```python
from build123d import *

# Parameters (mm, degrees)
SKETCH2_W           = 50
SKETCH2_H           = 53
BOSS_EXTRUDE1_DEPTH = 3
SKETCH3_W           = 50
SKETCH3_H           = 48
SKETCH3_R           = 11
BOSS_EXTRUDE2_DEPTH = 3
BOSS_EXTRUDE3_DEPTH = 3


with BuildPart() as part:
    # Sketch2 → Boss-Extrude1 (new body)
    with BuildSketch(Plane(origin=(0, 0, 0), x_dir=(1, 0, 0), z_dir=(0, 1, 0))):
        with Locations((25, 26.5)):
            Rectangle(SKETCH2_W, SKETCH2_H)
        with BuildLine():
            Line((7.9, 12), (7.9, 42))
            ThreePointArc((7.9, 42), (10, 44.1), (12.1, 42))
            Line((12.1, 42), (12.1, 12))
            ThreePointArc((12.1, 12), (10, 9.9), (7.9, 12))
        make_face(mode=Mode.SUBTRACT)
        with BuildLine():
            Line((42.1, 12), (42.1, 42))
            ThreePointArc((42.1, 42), (40, 44.1), (37.9, 42))
            Line((37.9, 42), (37.9, 12))
            ThreePointArc((37.9, 12), (40, 9.9), (42.1, 12))
        make_face(mode=Mode.SUBTRACT)
    extrude(amount=BOSS_EXTRUDE1_DEPTH)

    # Sketch3 → Boss-Extrude2 (add)
    with BuildSketch(Plane.XY):
        with Locations((25, 27)):
            Rectangle(SKETCH3_W, SKETCH3_H)
        with Locations((25, 30)):
            Circle(SKETCH3_R, mode=Mode.SUBTRACT)
    extrude(amount=-BOSS_EXTRUDE2_DEPTH)

    # Sketch4 → Boss-Extrude3 (add)
    with BuildSketch(Plane(origin=(50, 0, 0), x_dir=(0, 0, -1), z_dir=(1, 0, 0))):
        Polygon((16, 3), (3, 23), (3, 3), align=None)
    boss_extrude3 = extrude(amount=-BOSS_EXTRUDE3_DEPTH)

    # Mirror1: Boss-Extrude3 across plane
    add(boss_extrude3.mirror(Plane.ZY.offset(-25)))


solid = part.part
```
For this review, take the finished solid that the model builds, in its own axes (mm). A direction names the side the tool comes from. Round coordinates to 2 decimals unless told otherwise and drop trailing zeros. Write each loop counter-clockwise with the first axis right and the second up, starting at its lowest first coordinate (ties: lowest second). Pieces come first, ordered by that corner, then holes. Notation, with made-up numbers: (-33, 79) -> (-8, 79) arc R10 ccw to (-8, 86) -> close; hole circle Ø5 at (56.25, 38). An arc over 180 degrees is marked (long way). One line per question, with ' | ' between items. Start each with the question number.
1) Add section D-D (x = 25). Write out the cut boundary in (y, z), and give its area (3 significant figures).
2) Wall thickness on line 1 along Y through (x, z) = (25, -1); line 2 along Z through (x, y) = (33, 45); line 3 along X through (y, z) = (20, -1.5): over which ranges is each line inside the solid? List them lowest first.
3) Add section A-A (x = 10). Write out the cut boundary in (y, z), and give its area (3 significant figures).
4) Machinability: for faces 1 (the flat face through (25, 51, -1)), 2 (the cylindrical face through (10, 1.5, -9.9)), 3 (the flat face through (36, 27, -3)), which of the approach directions +Z, -Z, +X, -X, +Y, -Y give a long, thin tool a straight path to every point of the face, cutting with its end or side? Answer none if there is none.
5) Add section B-B (z = -22). Write out the cut boundary in (x, y), and give its area (3 significant figures).
6) Add section C-C (y = 27.5). Write out the cut boundary in (x, z), and give its area (3 significant figures).
7) For pin 1 Ø14.5 at (x, y) = (19, 32) entering from -Z; pin 2 Ø25 at (x, z) = (24.5, -28) entering from +Y, all flat-tipped, find the tip position at first contact; note any pin that passes through.
8) Mouldability with a two-part tool opening along Z and no side actions: class faces 4 (the flat face through (7.9, 1, -27)), 5 (the flat face through (48.52, 12.86, -9.59)), 6 (the flat face through (25, 3, -28)), 7 (the flat face through (37.9, 1, -27)) as +Z half, -Z half, draft (parallel to the pull), parting line (faces both ways), or undercut.
Reported:
1) outline: (0, -53) -> (3, -53) -> (3, -3) -> (19, -3) -> (19, 0) -> (0, 0) -> close; (41, -3) -> (51, -3) -> (51, 0) -> (41, 0) -> close | area: 237 mm²
2) line 1: y = 0 to 19, 41 to 51 | line 2: z = -3 to 0 | line 3: x = 0 to 20.42, 29.58 to 50
3) outline: (0, -53) -> (3, -53) -> (3, -44.1) -> (0, -44.1) -> close; (0, -9.9) -> (3, -9.9) -> (3, -3) -> (51, -3) -> (51, 0) -> (0, 0) -> close | area: 200 mm²
4) face 1: +Z, -Z, +X, -X, +Y | face 2: +Y, -Y | face 3: -Z, +Y
5) outline: (0, 0) -> (7.9, 0) -> (7.9, 3) -> (0, 3) -> close; (12.1, 0) -> (37.9, 0) -> (37.9, 3) -> (12.1, 3) -> close; (42.1, 0) -> (50, 0) -> (50, 3) -> (42.1, 3) -> close | area: 125 mm²
6) outline: (0, -3) -> (14.29, -3) -> (14.29, 0) -> (0, 0) -> close; (35.71, -3) -> (50, -3) -> (50, 0) -> (35.71, 0) -> close | area: 85.7 mm²
7) pin 1: stops at z = -3 | pin 2: stops at y = 3
8) face 4: undercut | face 5: -Z half | face 6: draft | face 7: undercut
